```python
from build123d import *

# Parameters (mm, degrees)
SKETCH1_W               = 50
SKETCH1_H               = 90
BOSS_EXTRUDE1_DEPTH     = 20
SKETCH2_W               = 20.25
SKETCH2_H               = 5.1
CUT_EXTRUDE1_DEPTH      = 1
CUT_EXTRUDE1_DEPTH_BACK = 51
SKETCH3_R               = 4.25
CUT_EXTRUDE2_DEPTH      = 21
CHAMFER1_SIZE           = 1
CHAMFER1_SIZE2          = 0.577350269
CHAMFER1_PART_2_SIZE    = 1
CHAMFER1_PART_2_SIZE2   = 0.577350269
CHAMFER1_PART_3_SIZE    = 1
CHAMFER1_PART_3_SIZE2   = 0.577350269
CHAMFER1_PART_4_SIZE    = 1
CHAMFER1_PART_4_SIZE2   = 0.577350269
CHAMFER2_SIZE           = 1


with BuildPart() as part:
    # Sketch1 → Boss-Extrude1 (new body)
    with BuildSketch(Plane(origin=(0, 0, 0), x_dir=(1, 0, 0), z_dir=(0, 1, 0))):
        Rectangle(SKETCH1_W, SKETCH1_H)
    extrude(amount=BOSS_EXTRUDE1_DEPTH)

    # Sketch2 → Cut-Extrude1 (cut, two sides)
    with BuildSketch(Plane(origin=(25, 0, 0), x_dir=(0, 0, -1), z_dir=(1, 0, 0))) as cut_extrude1_sk:
        with Locations((0, 2.55)):
            Rectangle(SKETCH2_W, SKETCH2_H)
    extrude(amount=CUT_EXTRUDE1_DEPTH, mode=Mode.SUBTRACT)
    extrude(cut_extrude1_sk.sketch, amount=-CUT_EXTRUDE1_DEPTH_BACK, mode=Mode.SUBTRACT)

    # Sketch3 → Cut-Extrude2 (cut, through all)
    with BuildSketch(Plane.XZ):
        with Locations((-15, 35)):
            Circle(SKETCH3_R)
        with Locations((-15, -35)):
            Circle(SKETCH3_R)
        with Locations((15, 35)):
            Circle(SKETCH3_R)
        with Locations((15, -35)):
            Circle(SKETCH3_R)
    extrude(amount=-CUT_EXTRUDE2_DEPTH, mode=Mode.SUBTRACT)

    # Chamfer1
    chamfer1_edges = [part.edges().sort_by_distance(p)[0] for p in [
        (-19.25, 20, 35),
    ]]
    chamfer1_side = [part.faces().sort_by_distance(p)[0] for p in [
        (-19.25, 10, 35),
    ]]
    chamfer(chamfer1_edges, length=CHAMFER1_SIZE, length2=CHAMFER1_SIZE2, reference=chamfer1_side[0])

    # Chamfer1 part 2
    chamfer1_part_2_edges = [part.edges().sort_by_distance(p)[0] for p in [
        (10.75, 20, 35),
    ]]
    chamfer1_part_2_side = [part.faces().sort_by_distance(p)[0] for p in [
        (10.75, 10, 35),
    ]]
    chamfer(chamfer1_part_2_edges, length=CHAMFER1_PART_2_SIZE, length2=CHAMFER1_PART_2_SIZE2, reference=chamfer1_part_2_side[0])

    # Chamfer1 part 3
    chamfer1_part_3_edges = [part.edges().sort_by_distance(p)[0] for p in [
        (10.75, 20, -35),
    ]]
    chamfer1_part_3_side = [part.faces().sort_by_distance(p)[0] for p in [
        (10.75, 10, -35),
    ]]
    chamfer(chamfer1_part_3_edges, length=CHAMFER1_PART_3_SIZE, length2=CHAMFER1_PART_3_SIZE2, reference=chamfer1_part_3_side[0])

    # Chamfer1 part 4
    chamfer1_part_4_edges = [part.edges().sort_by_distance(p)[0] for p in [
        (-19.25, 20, -35),
    ]]
    chamfer1_part_4_side = [part.faces().sort_by_distance(p)[0] for p in [
        (-19.25, 10, -35),
    ]]
    chamfer(chamfer1_part_4_edges, length=CHAMFER1_PART_4_SIZE, length2=CHAMFER1_PART_4_SIZE2, reference=chamfer1_part_4_side[0])

    # Chamfer2
    chamfer2_edges = [part.edges().sort_by_distance(p)[0] for p in [
        (0, 0, -10.125),
        (0, 0, 10.125),
    ]]
    chamfer(chamfer2_edges, length=CHAMFER2_SIZE)


solid = part.part
```
The listing builds one solid part. Answer for the finished solid, in the listing's coordinates (mm). A direction names the side the tool comes from. Give positions to 0.01 mm unless a question says otherwise; leave off trailing zeros. Order: outer loops, then holes, each group sorted by start corner. A loop starts at its lowest first (then second) coordinate and runs counter-clockwise, first axis right, second up.
1) Consider line 1 along Z through (x, y) = (15, 9.75); line 2 along Z through (x, y) = (-15, 4.5) (3 decimals); line 3 along X through (y, z) = (5.5, -32). Determine where each line is inside the solid, lowest interval first.
Reported:
line 1: z = -45 to -39.25, -30.75 to 30.75, 39.25 to 45
line 2: z = -45 to -39.25, -30.75 to -10.125, 10.125 to 30.75, 39.25 to 45
line 3: x = -25 to -18.01, -11.99 to 11.99, 18.01 to 25
2) Find section D-D on z = 35. Write down the section's boundary in (x, y).
Reported:
outline: (-25, 0) - (-19.25, 0) - (-19.25, 19) - (-19.83, 20) - (-25, 20) - close; (-10.75, 0) - (10.75, 0) - (10.75, 19) - (10.17, 20) - (-10.17, 20) - (-10.75, 19) - close; (19.25, 0) - (25, 0) - (25, 20) - (19.83, 20) - (19.25, 19) - close
3) Find section A-A on y = 3. Write down the section's boundary in (x, z) (3 decimals).
Reported:
outline: (-25, -45) - (25, -45) - (25, -10.125) - (-25, -10.125) - close; (-25, 10.125) - (25, 10.125) - (25, 45) - (-25, 45) - close; hole circle Ø8.5 at (-15, -35); hole circle Ø8.5 at (-15, 35); hole circle Ø8.5 at (15, -35); hole circle Ø8.5 at (15, 35)
4) Find section C-C on y = 16. Write down the section's boundary in (x, z).
Reported:
outline: (-25, -45) - (25, -45) - (25, 45) - (-25, 45) - close; hole circle Ø8.5 at (-15, -35); hole circle Ø8.5 at (-15, 35); hole circle Ø8.5 at (15, -35); hole circle Ø8.5 at (15, 35)
5) For faces 4 (the face through (0, 0, 28)), 5 (the face through (0, 3, 10.125)), determine the directions among +Z, -Z, +X, -X, +Y, -Y from which every point of the face is accessible in a straight line to the end or side of a thin tool.
Reported:
face 4: +Z, -Z, +X, -X, -Y
face 5: +X, -X, -Y
6) Find section B-B on x = -15. Write down the section's boundary in (y, z) (3 decimals), then the cut area to 3 significant figures.
Reported:
outline: (0, -45) - (20, -45) - (20, -39.827) - (19, -39.25) - (0, -39.25) - close; (0, -30.75) - (19, -30.75) - (20, -30.173) - (20, 30.173) - (19, 30.75) - (0, 30.75) - (0, 11.125) - (1, 10.125) - (5.1, 10.125) - (5.1, -10.125) - (1, -10.125) - (0, -11.125) - close; (0, 39.25) - (19, 39.25) - (20, 39.827) - (20, 45) - (0, 45) - close
area: 1,350 mm2
7) Given P1, Ø11, axis at x = -15, z = -35, coming from the +Y side; P2, Ø7.5, axis at x = -15, z = 35, coming from the -Y side; P3, Ø5, axis at x = -18, z = 6.5, coming from the -Y side, each flat-ended and moving along its own axis, determine where each tip first touches the part or whether it passes through.
Reported:
P1: stops at y = 20
P2: passes through
P3: stops at y = 5.1
8) Determine the mould class of faces 1 (the face through (14.447, 9.367, 39.214)), 2 (the face through (-25, 10, 1)), 3 (the face through (0, 10, 45)) for opening direction X: pulls with the +X half, pulls with the -X half, needs draft (parallel to the pull), parting line crosses it, or undercut.
Reported:
face 1: undercut
face 2: pulls with the -X half
face 3: needs draft
